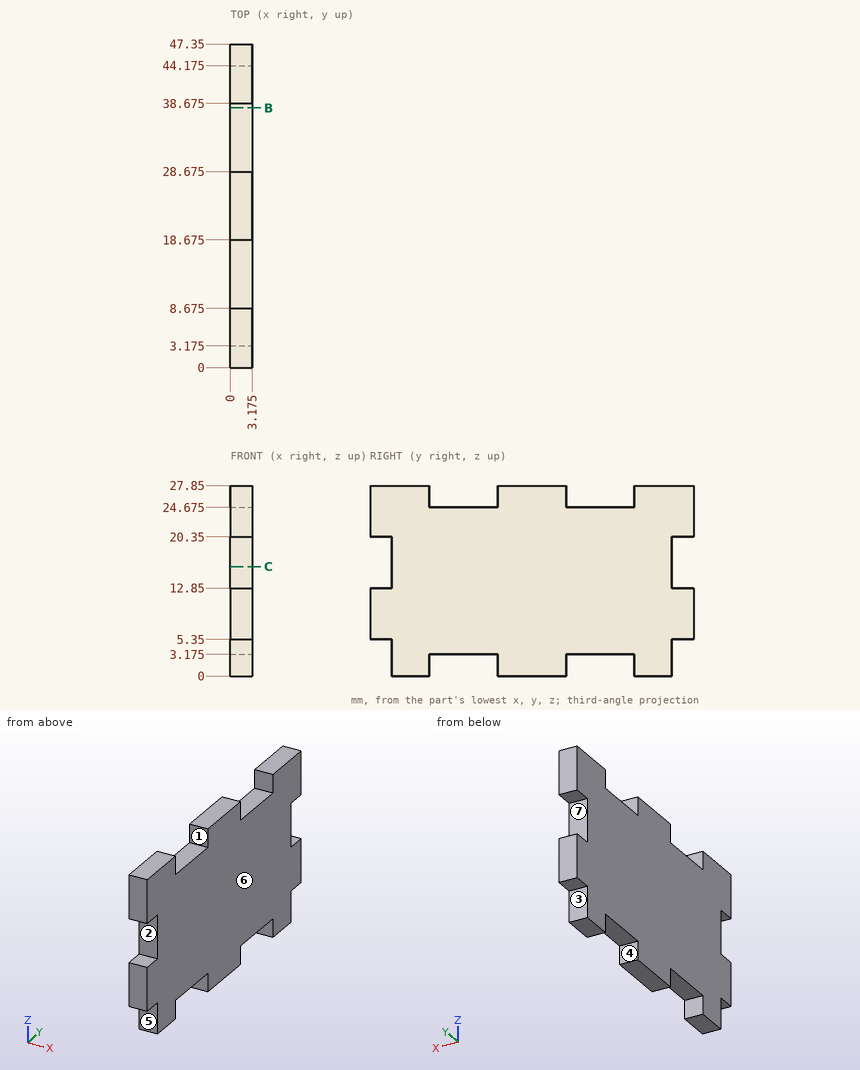
Verification items for this drawing (mm, ordinates from the low corner). A direction names the side the tool comes from. Coordinates: 2 decimals unless noted, no trailing zeros. Order: outer loops, then holes, each group sorted by start corner. A loop starts at its lowest first (then second) coordinate and runs counter-clockwise, first axis right, second up. Notation, with made-up numbers: (77, -31.75) - (104, -31.75) arc R19 ccw to (104, -26.75) - close; hole circle Ø5 at (16.5, 31). An arc over 180 degrees is marked (long way). Answer as a JSON object with one key per item and string values. Group by question number.
Item 1: Sectioned sample at C-C, the plane z = 16. Record the cut outline in (x, y) (3 decimals).
Item 2: Scan lines: probe 1 along Y at (x, z) = (2.3, 25) (3 decimals); probe 2 along Z at (x, y) = (1.5, 29.5) (3 decimals); probe 3 along Y at (x, z) = (2, 20.25) (3 decimals). Record each from-to range of solid material in increasing order.
Item 3: Depth check by flat-ended pin: pin 1 Ø1 at (x, y) = (2, 46) entering from -Z; pin 2 Ø1 at (x, z) = (1, 2.5) entering from +Y (3 decimals); pin 3 Ø4 at (y, z) = (9, 21.5) entering from -X; pin 4 Ø1.6 at (x, y) = (1.5, 14.5) entering from -Z (3 decimals). Enter the tip coordinate at first touch or a pass-through.
Item 4: Draft check along Z on the marked faces 6 and 7. Enter one of: +Z half, -Z half, draft (parallel to the pull), parting line (faces both ways), or undercut.
Item 5: Sectioned sample at B-B, the plane y = 38. Record the cut outline in (x, z) (3 decimals).
Item 6: Tool access check on the marked faces 1, 2, 3, 4 and 5. Record the directions out of +Z, -Z, +X, -X, +Y, -Y that give a thin tool (end or side, any length) a straight path to the whole face; none if there is none.
Resolved:
{
 "1": {"outline": "(0, 3.175) - (3.175, 3.175) - (3.175, 44.175) - (0, 44.175) - close"},
 "2": {"probe 1": "0 to 8.675, 18.675 to 28.675, 38.675 to 47.35", "probe 2": "3.175 to 24.675", "probe 3": "3.175 to 44.175"},
 "3": {"pin 1": "z = 5.35", "pin 2": "y = 44.175", "pin 3": "x = 0", "pin 4": "z = 3.175"},
 "4": {"face 6": "draft", "face 7": "undercut"},
 "5": {"outline": "(0, 3.175) - (3.175, 3.175) - (3.175, 24.675) - (0, 24.675) - close"},
 "6": {"face 1": "+Z, +X, -X", "face 2": "+X, -X, -Y", "face 3": "-Z, +X, -X, +Y", "face 4": "-Z, +X, -X", "face 5": "-Z, +X, -X, -Y"}
}
